Design review of the part built by this model. Coordinates are the model's own, in mm. A direction names the side the tool comes from. Round coordinates to 2 decimals unless told otherwise and drop trailing zeros. Loops run counter-clockwise (first coordinate to the right, second up) from the corner with the lowest first, then second, coordinate; pieces in that order, holes last. Notation, with made-up numbers: (27.5, 60) - (49.5, 60) arc R26 cw to (49.5, 83) - close; hole circle Ø11 at (89, -16.75). An arc over 180 degrees is marked (long way). Answer as CSV lines item,"result". Start each with the question number.
(1) For faces 5 (the flat face through (770, 819, 683)), 6 (the flat face through (394, 1660, 744)), list the 3-axis set-ups (+Z, -Z, +X, -X, +Y, -Y) from which the entire face can be reached by the end or side of a thin tool; tool diameter is ignored.
(2) Consider section D-D (z = 494). Give the boundary of the cut face in (x, y).
(3) For P1, Ø6, axis at x = 240, y = 1005, coming from the -Z side; P2, Ø9, axis at x = 17, y = 967, coming from the -Z side; P3, Ø12, axis at x = 516, y = 223.5, coming from the +Z side, all flat-tipped, find the tip position at first contact; note any pin that passes through.
(4) Consider section A-A (x = 748). Give the boundary of the cut face in (y, z).
(5) Consider section C-C (y = 211). Give the boundary of the cut face in (x, z).
(6) Mouldability with a two-part tool opening along X and no side actions: class faces 1 (the flat face through (0, 818, 744)), 2 (the flat face through (394, 0, 744)), 3 (the flat face through (800, 818, 744)), 4 (the flat face through (30, 819, 683)) as released by +X, released by -X, zero draft, split by the parting line, or undercut.
(7) Wall thickness on L1, parallel to X at y = 1392, z = 840; L2, parallel to Y at x = 277.5, z = 790.5; L3, parallel to Z at x = 525, y = 452.5: over which ranges is each line inside the solid? List them lowest first.
(8) Consider section B-B (z = 292.5). Give the boundary of the cut face in (x, y), and give its area (3 significant figures).
from build123d import *

# Parameters (mm, degrees)
F0_W     = 1600
F0_H     = 290
F1_DEPTH = 800
F3_DEPTH = 500.001
F4_W     = 740
F4_H     = 150
F4_H_2   = 290
F5_DEPTH = 1660.001
F6_W     = 800
F6_H     = 1660
F6_W_2   = 740
F6_H_2   = 1600
F7_DEPTH = 400
F8_W     = 770
F8_H     = 1660
F9_DEPTH = 2


with BuildPart() as f1:
    # F0 (on Right) → F1 (new body)
    with BuildSketch(Plane.YZ):
        Polygon((0, 500), (0, 0), (30, 0), (30, 150), (1630, 150), (1630, 0), (1660, 0), (1660, 500), align=None)
        with Locations((830, 325)):
            Rectangle(F0_W, F0_H, mode=Mode.SUBTRACT)
    extrude(amount=F1_DEPTH)

    # F2 (on face) → F3 (cut, through all)
    with BuildSketch(Plane.XY.offset(500)):
        Polygon((30, 30), (770, 30), (770, 1630), (385, 1630), (30, 1630), align=None)
    extrude(amount=-F3_DEPTH, mode=Mode.SUBTRACT)

    # F4 (on face) → F5 (cut, through all)
    with BuildSketch(Plane(origin=(0, 1660, 0), x_dir=(-1, 0, 0), z_dir=(0, 1, 0))):
        with Locations((-400, 75)):
            Rectangle(F4_W, F4_H)
        with Locations((-400, 325)):
            Rectangle(F4_W, F4_H_2)
    extrude(amount=-F5_DEPTH, mode=Mode.SUBTRACT)

    # F6 (on face) → F7 (join)
    with BuildSketch(Plane.XY.offset(500)):
        with Locations((400, 830)):
            Rectangle(F6_W, F6_H)
        with Locations((400, 830)):
            Rectangle(F6_W_2, F6_H_2, mode=Mode.SUBTRACT)
    extrude(amount=F7_DEPTH)

    # F8 (on face) → F9 (join)
    with BuildSketch(Plane(origin=(0, 0, 470), x_dir=(1, 0, 0), z_dir=(0, 0, -1))):
        with Locations((385, -830)):
            Rectangle(F8_W, F8_H)
    extrude(amount=-F9_DEPTH)


solid = f1.part
Determined:
1,face 5,"+Z"
1,face 6,"+Z, -Z, +X, -X, +Y"
2,outline,"(0, 0) - (800, 0) - (800, 1660) - (0, 1660) - close; hole (30, 30) - (770, 30) - (770, 1630) - (30, 1630) - close"
3,P1,"stops at z = 470"
3,P2,"stops at z = 150"
3,P3,"stops at z = 472"
4,outline,"(0, 150) - (30, 150) - (30, 180) - (0, 180) - close; (0, 470) - (1660, 470) - (1660, 900) - (1630, 900) - (1630, 472) - (30, 472) - (30, 900) - (0, 900) - close; (1630, 150) - (1660, 150) - (1660, 180) - (1630, 180) - close"
5,outline,"(0, 150) - (30, 150) - (30, 180) - (0, 180) - close; (0, 470) - (800, 470) - (800, 900) - (770, 900) - (770, 472) - (30, 472) - (30, 900) - (0, 900) - close; (770, 150) - (800, 150) - (800, 180) - (770, 180) - close"
6,face 1,"released by -X"
6,face 2,"zero draft"
6,face 3,"released by +X"
6,face 4,"undercut"
7,L1,"x = 0 to 30, 770 to 800"
7,L2,"y = 0 to 30, 1630 to 1660"
7,L3,"z = 470 to 472"
8,outline,"(0, 0) - (30, 0) - (30, 30) - (0, 30) - close; (0, 1630) - (30, 1630) - (30, 1660) - (0, 1660) - close; (770, 0) - (800, 0) - (800, 30) - (770, 30) - close; (770, 1630) - (800, 1630) - (800, 1660) - (770, 1660) - close"
8,area,"3,600 mm^2"
